For this review, take the finished solid that the model builds, in its own axes (mm). A direction names the side the tool comes from. Coordinates: 2 decimals unless noted, no trailing zeros. Order: outer loops, then holes, each group sorted by start corner. A loop starts at its lowest first (then second) coordinate and runs counter-clockwise, first axis right, second up. Notation, with made-up numbers: (1, -9) -> (8, -9) arc R13 cw to (8, 10) -> close; hole circle Ø9 at (65.5, 15.25). An arc over 180 degrees is marked (long way). Return JSON: item names as keys, results as strings. Group by question number.
Item 1: Machinability: for faces 1 (the flat face through (-18, 3, 1)), 2 (the cylindrical face through (9.301, 11.715, 0.105)), 3 (the flat face through (10, 5, 0)), 4 (the flat face through (-13, 6, 0)), 5 (the flat face through (-18, 3, -1)), which of the approach directions +Z, -Z, +X, -X, +Y, -Y give a long, thin tool a straight path to every point of the face, cutting with its end or side? Answer none if there is none.
Item 2: For line 1 along X through (y, z) = (3, 4.75); line 2 along Y through (x, z) = (3, 2.75); line 3 along X through (y, z) = (-1.5, 1.25), list the stretches that pass through material, from the lowest coordinate up.
Item 3: Draft analysis for pull direction X (two halves, no side actions). For faces 6 (the flat face through (-1, 12, 0)), 7 (the flat face through (-13, 2, 0)), 8 (the cylindrical face through (-34, -4, 0)), state which applies: +X half, -X half, draft (parallel to the pull), parting line (faces both ways), or undercut.
Item 4: Take a section at B-B (z = 4.25). Write out the cut boundary in (x, y), then the cut area to 3 significant figures.
Item 5: Take a section at D-D (x = -10.5). Write out the cut boundary in (y, z), then the cut area to 3 significant figures.
Item 6: Take a section at C-C (y = 3.25). Write out the cut boundary in (x, z), then the cut area to 4 significant figures.
Item 7: Take a section at A-A (y = -1). Write out the cut boundary in (x, z).
Item 8: Insertion check: pin 1 (4 mm diameter, centred on x = 3, z = 5.5, fed in from -Y); pin 2 (2 mm diameter, centred on x = -10.5, z = 0.5, fed in from -Y); pin 3 (2 mm diameter, centred on x = -12, z = 0, fed in from +Y); pin 4 (6 mm diameter, centred on x = -17.5, y = -2, fed in from +Z). Each pin has a flat end and moves straight along its axis. Give the tip position at first contact, or say it passes through.
```python
from build123d import *

# Parameters (mm, degrees)
PAD_DEPTH    = 7.5
SKETCH001_W  = 4
SKETCH001_H  = 2
PAD001_DEPTH = 24
PAD002_DEPTH = 1


with BuildPart() as part:
    # Sketch → Pad (new body, symmetric)
    with BuildSketch(Plane.XY):
        with BuildLine():
            Line((0, 0), (10, 0))
            Line((10, 0), (10, 10))
            Line((10, 10), (9, 10))
            Line((9, 11), (9, 10))
            ThreePointArc((10, 12), (9.292893, 11.707107), (9, 11))
            Line((10, 12), (12, 12))
            Line((12, 12), (12, -2))
            Line((12, -2), (-2, -2))
            Line((-2, 12), (-2, -2))
            Line((0, 12), (-2, 12))
            Line((0, 0), (0, 12))
        make_face()
    extrude(amount=PAD_DEPTH, both=True)

    # Sketch001 → Pad001 (join)
    with BuildSketch(Plane.YZ):
        with Locations((4, 0)):
            Rectangle(SKETCH001_W, SKETCH001_H)
    extrude(amount=-PAD001_DEPTH)

    # Sketch002 → Pad002 (join, symmetric)
    with BuildSketch(Plane.XY):
        with BuildLine():
            Line((-24, 6), (-32, -2))
            ThreePointArc((-32, -2), (-34, -4), (-32, -6))
            Line((-32, -6), (-24, 2))
            Line((-24, 2), (-24, 6))
        make_face()
    extrude(amount=PAD002_DEPTH, both=True)


solid = part.part
```
Findings below:
{
 "1": {"face 1": "+Z, -X, +Y, -Y", "face 2": "+Z, -Z, +Y", "face 3": "+Z, -Z", "face 4": "+Z, -Z, -X, +Y", "face 5": "-Z, -X, +Y, -Y"},
 "2": {"line 1": "x = -2 to 0, 10 to 12", "line 2": "y = -2 to 0", "line 3": "x = -2 to 12"},
 "3": {"face 6": "draft", "face 7": "undercut", "face 8": "-X half"},
 "4": {"outline": "(-2, -2) -> (12, -2) -> (12, 12) -> (10, 12) arc R1 ccw to (9, 11) -> (9, 10) -> (10, 10) -> (10, 0) -> (0, 0) -> (0, 12) -> (-2, 12) -> close", "area": "77.8 mm2"},
 "5": {"outline": "(2, -1) -> (6, -1) -> (6, 1) -> (2, 1) -> close", "area": "8.00 mm2"},
 "6": {"outline": "(-26.75, -1) -> (-2, -1) -> (-2, -7.5) -> (0, -7.5) -> (0, 7.5) -> (-2, 7.5) -> (-2, 1) -> (-26.75, 1) -> close; (10, -7.5) -> (12, -7.5) -> (12, 7.5) -> (10, 7.5) -> close", "area": "109.5 mm2"},
 "7": {"outline": "(-31, -1) -> (-27, -1) -> (-27, 1) -> (-31, 1) -> close; (-2, -7.5) -> (12, -7.5) -> (12, 7.5) -> (-2, 7.5) -> close"},
 "8": {"pin 1": "stops at y = -2", "pin 2": "stops at y = 2", "pin 3": "stops at y = 6", "pin 4": "passes through"}
}
